Can you work these out from the model? Positions are in its coordinate system, mm. A direction names the side the tool comes from. Round coordinates to 2 decimals unless told otherwise and drop trailing zeros. Write each loop counter-clockwise with the first axis right and the second up, starting at its lowest first coordinate (ties: lowest second). Pieces come first, ordered by that corner, then holes. Notation, with made-up numbers: M 78.25,44 L 119.25,44 A26 cw 119.25,70 Z; hole C 48,-1.5 d1. An arc over 180 degrees is marked long. Answer in a Markdown table with one row per item. Add a question column.
(1) Suppose I cut it at C-C, the plane x = 60.5. Write out the boundary of the cut face in (y, z), then the cut area to 3 significant figures.
(2) If we mould it in two halves opening along Y, with no side actions, what happens to faces 1 (the face through (23.1, 16.8, 23.14)), 2 (the face through (66.516, 3.011, 3.65)), 3 (the face through (37.188, 15.571, 26.465))? For each: released by +Y, released by -Y, zero draft, split by the parting line, or undercut.
(3) Suppose I cut it at D-D, the plane y = 24. Write out the boundary of the cut face in (x, z), then the cut area to 3 significant figures.
(4) Suppose I cut it at A-A, the plane x = 46. Write out the boundary of the cut face in (y, z), then the cut area to 3 significant figures.
(5) If I drill on probe 1 along Y at (x, z) = (-15.5, 27.95); probe 2 along X at (y, z) = (4, 15); probe 3 along X at (y, z) = (4, 15.5), over which ranges is the centre line in solid material (lowest first)?
(6) For faces 4 (the face through (61, 5, 21)), 5 (the face through (30.33, 35.16, -0.29)), 6 (the face through (0, 29, 24)), 7 (the face through (-14.42, 2.46, -16.68)), 8 (the face through (43, 20, 0)), which set-ups out of +Z, -Z, +X, -X, +Y, -Y let a thin tool reach every point of the face, with its end or its side?
(7) Suppose I cut it at B-B, the plane z = 0. Write out the boundary of the cut face in (x, y), then the cut area to 3 significant figures.
(8) I'm going to push flat-ended pins straight in: pin 1 (12 mm diameter, centred on x = 13.5, y = 24.5, fed in from -Z); pin 2 (4 mm diameter, centred on x = 15.5, z = -15.5, fed in from +Y); pin 3 (5 mm diameter, centred on y = 20.5, z = -15, fed in from +X). Where does each tip first touch, or does it pass through?
from build123d import *

# Parameters (mm, degrees)
SKETCH_1_R          = 1.6
SKETCH_1_R_2        = 12
EXTRUDE_1_DEPTH     = 5
SKETCH_4_W          = 45
SKETCH_4_H          = 50
SKETCH_4_R          = 1.6
EXTRUDE_4_DEPTH     = 5
SKETCH_5_W          = 50
SKETCH_5_H          = 50
EXTRUDE_5_DEPTH     = 50
SKETCH_6_R          = 2.4
SKETCH_6_R_2        = 1.9
CUT_EXTRUDE_1_DEPTH = 103.352332655
SKETCH_7_R          = 1.8
CUT_EXTRUDE_2_DEPTH = 94.898881782
SKETCH_8_R          = 2.8
CUT_EXTRUDE_3_DEPTH = 45
SKETCH_9_W          = 17
SKETCH_9_H          = 20
CUT_EXTRUDE_4_DEPTH = 45
CHAMFER_1_SIZE      = 50
FILLET_1_R          = 5
FILLET_4_R          = 10
FILLET_5_R          = 25
FILLET_6_R          = 3
FILLET_7_R          = 1.5


with BuildPart() as part:
    # 草图1 → 凸台-拉伸1 (new body)
    with BuildSketch(Plane(origin=(0, 0, 0), x_dir=(1, 0, 0), z_dir=(0, 1, 0))):
        Polygon((24, -24), (24, 21), (21, 21), (-21, 21), (-21, -21), (-21, -24), align=None)
        with Locations(Location((-15.5, 15.5, 0), (0, 0, 270))):
            Circle(SKETCH_1_R, mode=Mode.SUBTRACT)
        with Locations(Location((15.5, 15.5, 0), (0, 0, 270))):
            Circle(SKETCH_1_R, mode=Mode.SUBTRACT)
        with Locations(Location((-15.5, -15.5, 0), (0, 0, 270))):
            Circle(SKETCH_1_R, mode=Mode.SUBTRACT)
        with Locations(Location((15.5, -15.5, 0), (0, 0, 270))):
            Circle(SKETCH_1_R, mode=Mode.SUBTRACT)
        with Locations(Location((0, 0, 0), (0, 0, 270))):
            Circle(SKETCH_1_R_2, mode=Mode.SUBTRACT)
    extrude(amount=EXTRUDE_1_DEPTH)

    # 草图4 → 凸台-拉伸4 (add)
    with BuildSketch(Plane.XY.offset(24)):
        with Locations((1.5, 25)):
            Rectangle(SKETCH_4_W, SKETCH_4_H)
        with Locations((-15.5, 44.5)):
            Circle(SKETCH_4_R, mode=Mode.SUBTRACT)
        with Locations((15.5, 44.5)):
            Circle(SKETCH_4_R, mode=Mode.SUBTRACT)
        with Locations((-15.5, 13.5)):
            Circle(SKETCH_4_R, mode=Mode.SUBTRACT)
        with Locations((15.5, 13.5)):
            Circle(SKETCH_4_R, mode=Mode.SUBTRACT)
    extrude(amount=EXTRUDE_4_DEPTH)

    # 草图5 → 凸台-拉伸5 (add)
    with BuildSketch(Plane(origin=(24, 0, 0), x_dir=(0, 0, -1), z_dir=(1, 0, 0))):
        with Locations((-4, 25)):
            Rectangle(SKETCH_5_W, SKETCH_5_H)
    extrude(amount=EXTRUDE_5_DEPTH)

    # 草图6 → 切除-拉伸1 (cut, through all)
    with BuildSketch(Plane(origin=(0, 0, -21), x_dir=(-1, 0, 0), z_dir=(0, 0, -1))):
        with Locations((-46, 5)):
            Circle(SKETCH_6_R)
        with Locations((-46, 15)):
            Circle(SKETCH_6_R)
        with Locations((-39, 15)):
            Circle(SKETCH_6_R_2)
    extrude(amount=-CUT_EXTRUDE_1_DEPTH, mode=Mode.SUBTRACT)

    # 草图7 → 切除-拉伸2 (cut, through all)
    with BuildSketch(Plane.XZ):
        with Locations(Location((60.5, 19, 0), (0, 0, 270))):
            Circle(SKETCH_7_R)
    extrude(amount=-CUT_EXTRUDE_2_DEPTH, mode=Mode.SUBTRACT)

    # 草图8 → 切除-拉伸3 (cut)
    with BuildSketch(Plane(origin=(0, 50, 0), x_dir=(1, 0, 0), z_dir=(0, 1, 0))):
        with Locations(Location((60.5, -19, 0), (0, 0, 270))):
            Circle(SKETCH_8_R)
    extrude(amount=-CUT_EXTRUDE_3_DEPTH, mode=Mode.SUBTRACT)

    # 草图9 → 切除-拉伸4 (cut)
    with BuildSketch(Plane(origin=(0, 0, -21), x_dir=(-1, 0, 0), z_dir=(0, 0, -1))):
        with Locations((-42.5, 10)):
            Rectangle(SKETCH_9_W, SKETCH_9_H)
    extrude(amount=-CUT_EXTRUDE_4_DEPTH, mode=Mode.SUBTRACT)

    # 倒角1
    # the kernel refuses this chamfer: 50 mm, written as the material it takes off along each edge
    with BuildSketch(Plane(origin=(74, 50, 157.584149398), x_dir=(-0.9996219169112969, 0.027495876610586317, 0), z_dir=(0, 0, -1))) as chamfer_1_piece_1:
        Polygon((CHAMFER_1_SIZE * 0.999621916911, -CHAMFER_1_SIZE * 0.0274958766106), (-CHAMFER_1_SIZE * 0.0274958766106, -CHAMFER_1_SIZE * 0.999621916911), (0, 0), align=None)
    extrude(amount=307.168298797, mode=Mode.SUBTRACT)

    # 圆角1
    # the kernel refuses this fillet: 5 mm, written as the material it takes off along each edge
    with BuildSketch(Plane(origin=(74, 0, -51.17766953), x_dir=(-0.707106781186265, 0.7071067811868301, 0), z_dir=(0, 0, 1))) as fillet_1_piece_1:
        with BuildLine():
            CenterArc((FILLET_1_R * 2.41421356237, FILLET_1_R), FILLET_1_R, 135, 135)
            Line((FILLET_1_R * 1.70710678118, FILLET_1_R * 1.70710678119), (0, 0))
            Line((0, 0), (FILLET_1_R * 2.41421356237, 0))
        make_face()
    extrude(amount=110.355339059, mode=Mode.SUBTRACT)

    # 圆角4
    fillet_4_edges = [part.edges().sort_by_distance(p)[0] for p in [
        (24, 50, 1.5),
    ]]
    fillet(fillet_4_edges, radius=FILLET_4_R)

    # 圆角5
    fillet_5_edges = [part.edges().sort_by_distance(p)[0] for p in [
        (24, 50, 26.5),
    ]]
    fillet(fillet_5_edges, radius=FILLET_5_R)

    # 圆角6
    fillet_6_edges = [part.edges().sort_by_distance(p)[0] for p in [
        (30.173165676, 35.096659701, 24),
        (24, 15.428932188, 24),
        (1.5, 5, 24),
        (24, 5, 1.5),
        (34, 20, 1.5),
        (51, 20, 1.5),
    ]]
    fillet(fillet_6_edges, radius=FILLET_6_R)

    # 圆角7
    fillet_7_edges = [part.edges().sort_by_distance(p)[0] for p in [
        (51, 8.5, 24),
        (42.5, 20, 24),
        (34, 8.5, 24),
        (50.121320344, 19.121320344, 24),
        (34.878679656, 19.121320344, 24),
    ]]
    fillet(fillet_7_edges, radius=FILLET_7_R)


solid = part.part
Calculated:
| question | item | result |
|---|---|---|
| 1 | outline | M 0,-21 L 13.5,-21 L 13.5,16.2 L 5,16.2 L 5,17.2 L 0,17.2 Z; M 0,20.8 L 5,20.8 L 5,21.8 L 13.5,21.8 L 13.5,29 L 0,29 Z |
| 1 | area | 609 mm² |
| 2 | face 1 | zero draft |
| 2 | face 2 | split by the parting line |
| 2 | face 3 | undercut |
| 3 | outline | M -21,24 L 21,24 A3 cw 24,21 L 24,-21 L 50,-21 L 50,29 L -21,29 Z |
| 3 | area | 1,530 mm² |
| 4 | outline | M 0,24 L 2.6,24 L 2.6,29 L 0,29 Z; M 7.4,24 L 12.6,24 L 12.6,29 L 7.4,29 Z; M 17.4,24 L 18.5,24 A1.5 cw 20,22.5 L 20,-21 L 28,-21 L 28,29 L 17.4,29 Z |
| 4 | area | 452 mm² |
| 5 | probe 1 | 0 to 11.9, 15.1 to 42.9, 46.1 to 50 |
| 5 | probe 2 | -21 to -17.02, -13.98 to 13.98, 17.02 to 34, 51 to 66.83 |
| 5 | probe 3 | -21 to -17.1, -13.9 to 13.9, 17.1 to 34, 51 to 66.83 |
| 6 | face 4 | +Y |
| 6 | face 5 | -Z, +Y |
| 6 | face 6 | -Z, -X, +Y |
| 6 | face 7 | +Y, -Y |
| 6 | face 8 | -Z, -Y |
| 7 | outline | M -21,0 L -12,0 L -12,5 L -21,5 Z; M 12,0 L 34,0 L 34,17 A3 cw 37,20 L 48,20 A3 cw 51,17 L 51,0 L 61.93,0 A5 ccw 65.46,8.54 L 41.07,32.93 A10 ccw 24,25.86 L 24,8 A3 cw 21,5 L 12,5 Z |
| 7 | area | 866 mm² |
| 8 | pin 1 | z = 24 |
| 8 | pin 2 | y = 5 |
| 8 | pin 3 | x = 56 |
